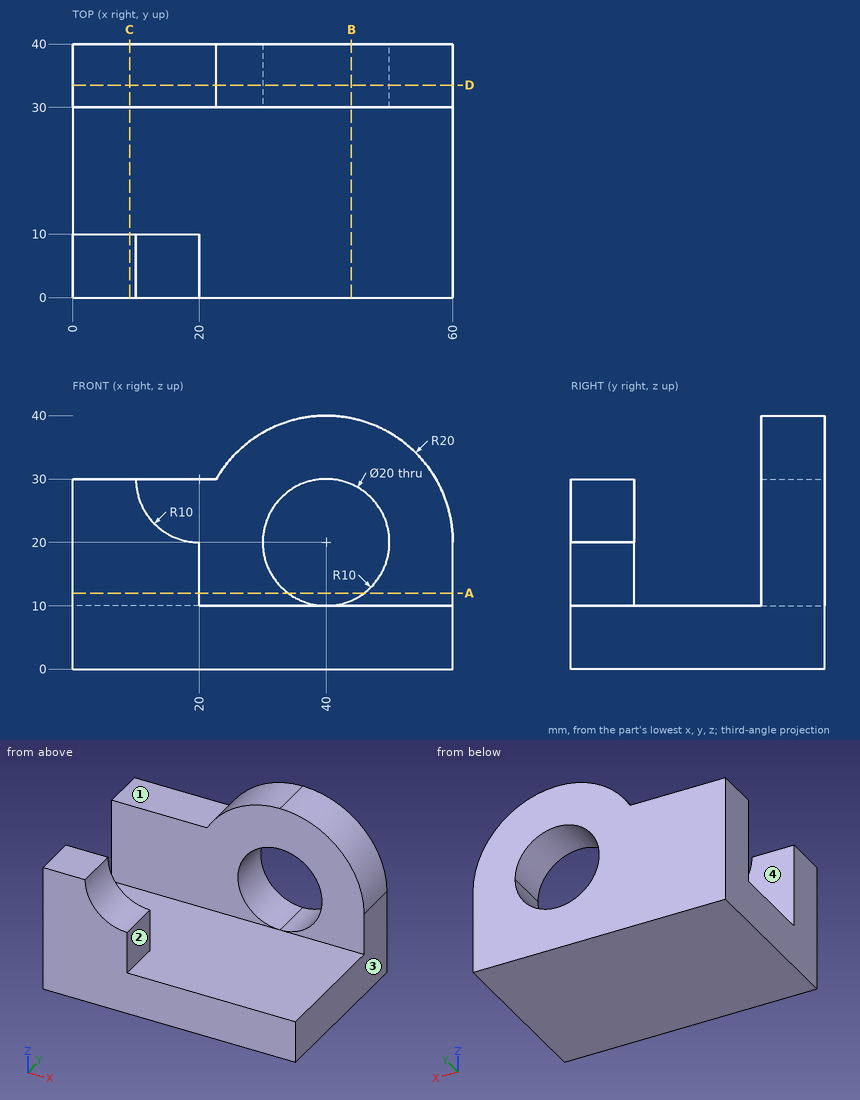
Input: dimensioned drawing with shaded views. Units: mm. Origin: part minimum x, y, z. A direction names the side the tool comes from. Round coordinates to 2 decimals unless told otherwise and drop trailing zeros. Loops run counter-clockwise (first coordinate to the right, second up) from the corner with the lowest first, then second, coordinate; pieces in that order, holes last.
1) Set-up query: the marked faces 1, 2, 3 and 4. Return all of +Z, -Z, +X, -X, +Y, -Y with unobstructed straight access to the full face (end or side cutting, diameter ignored); none if empty.
Ans:
face 1: +Z, -X, +Y, -Y
face 2: +Z, +X, -Y
face 3: +Z, -Z, +X, +Y, -Y
face 4: +Z, +X, -X
2) Section query A-A on z = 12. Return the cut outline in (x, y).
Ans:
outline: (0, 0) - (20, 0) - (20, 10) - (0, 10) - close; (0, 30) - (34, 30) - (34, 40) - (0, 40) - close; (46, 30) - (60, 30) - (60, 40) - (46, 40) - close
3) Material intervals for line 1 (Y direction, x = 10.5, z = 20); line 2 (X direction, y = 37, z = 20), sorted ascending.
Ans:
line 1: y = 0 to 10, 30 to 40
line 2: x = 0 to 30, 50 to 60
4) Section query B-B on x = 44. Return the cut outline in (y, z), plus the area to 3 significant figures.
Ans:
outline: (0, 0) - (40, 0) - (40, 10.83) - (30, 10.83) - (30, 10) - (0, 10) - close; (30, 29.17) - (40, 29.17) - (40, 39.6) - (30, 39.6) - close
area: 513 mm2
5) Pin query (flat end, axial travel): pin 1 (11 mm diameter, centred on x = 11, y = 37, fed in from +Z); pin 2 (4 mm diameter, centred on x = 23, y = 7.5, fed in from +Z); pin 3 (10 mm diameter, centred on y = 8, z = 29.5, fed in from +X). Return the tip coordinate at first contact, or that it passes through.
Ans:
pin 1: stops at z = 30
pin 2: stops at z = 10
pin 3: stops at x = 11.65
6) Section query C-C on x = 9. Return the cut outline in (y, z), plus the area to 3 significant figures.
Ans:
outline: (0, 0) - (40, 0) - (40, 30) - (30, 30) - (30, 10) - (10, 10) - (10, 30) - (0, 30) - close
area: 800 mm2
7) Section query D-D on y = 33.5. Return the cut outline in (x, z).
Ans:
outline: (0, 0) - (60, 0) - (60, 20) arc R20 ccw to (40, 40) arc R20 ccw to (22.68, 30) - (0, 30) - close; hole circle Ø20 at (40, 20)
